Here's how the part is built. I have some questions about the finished solid (model axes, mm). A direction names the side the tool comes from. Give positions to 0.01 mm unless a question says otherwise; leave off trailing zeros. Write each loop counter-clockwise with the first axis right and the second up, starting at its lowest first coordinate (ties: lowest second). Pieces come first, ordered by that corner, then holes. Notation, with made-up numbers: (-15, 52.5) -> (15, 52.5) arc R30 ccw to (15, 79.5) -> close; hole circle Ø1 at (30, -24). An arc over 180 degrees is marked (long way). Use CSV: the item, a comma, the result in double quotes. Start each with the question number.
(1) If we mould it in two halves opening along Y, with no side actions, what happens to faces 3 (the flat face through (-38.1, -26, 0)), 4 (the flat face through (-1, 38.1, 26)), 5 (the flat face through (24, 0, 22.893)), 6 (the flat face through (-25, 0, 22.893))? For each: pulls with the +Y half, pulls with the -Y half, needs draft (parallel to the pull), parting line crosses it, or undercut.
(2) Suppose I cut it at A-A on y = -17.5. List the corners of the cut face in (x, z) for me.
(3) I need wall thicknesses on L1, parallel to Z at x = 1, y = -18.5; L2, parallel to Z at x = 13, y = -9.5; L3, parallel to Y at x = -14, z = -24. Which ranges of each line are inside material? Lowest first, please. Write a range as [from, to].
(4) Which directions (+Z, -Z, +X, -X, +Y, -Y) give clear straight access to the entire face, cutting with the end or side of a thin tool? Please do faces 1 (the flat face through (-1, 0, -27.907)), 2 (the flat face through (0, -1, -38.1)).
(5) Suppose I cut it at C-C on x = 0. List the corners of the cut face in (y, z) for me, plus the area to 3 significant figures.
(6) Suppose I cut it at B-B on z = 0. List the corners of the cut face in (x, y) for me, plus the area to 3 significant figures.
(7) Suppose I cut it at D-D on y = -29.5. List the corners of the cut face in (x, z) for me, plus the area to 3 significant figures.
from build123d import *

# Parameters (mm, degrees)
F0_W     = 76.2
F0_H     = 76.2
F1_DEPTH = 38.1
F2_R     = 25.4
F3_DEPTH = 76.2
F4_R     = 5.08
F5_SIZE  = 5.08
F6_R     = 5.08
F7_R     = 5.08
F8_W     = 50.8
F8_H     = 50.8
F9_DEPTH = 76.2


with BuildPart() as f1:
    # F0 (on Front) → F1 (new body, symmetric)
    with BuildSketch(Plane.XZ):
        Rectangle(F0_W, F0_H)
    extrude(amount=F1_DEPTH, both=True)

    # F2 (on face) → F3 (cut)
    with BuildSketch(Plane.XZ.offset(38.1)):
        Circle(F2_R)
    extrude(amount=-F3_DEPTH, mode=Mode.SUBTRACT)

    # F4
    f4_edges = [f1.edges().sort_by_distance(p)[0] for p in [
        (38.1, 0, 38.1),
    ]]
    fillet(f4_edges, radius=F4_R)

    # F5
    f5_edges = [f1.edges().sort_by_distance(p)[0] for p in [
        (-38.1, 0, 38.1),
    ]]
    chamfer(f5_edges, length=F5_SIZE)

    # F6
    f6_edges = [f1.edges().sort_by_distance(p)[0] for p in [
        (38.1, 0, -38.1),
    ]]
    fillet(f6_edges, radius=F6_R)

    # F7
    f7_edges = [f1.edges().sort_by_distance(p)[0] for p in [
        (-38.1, 0, -38.1),
    ]]
    fillet(f7_edges, radius=F7_R)

    # F8 (on face) → F9 (cut)
    with BuildSketch(Plane(origin=(-38.1, 0, 0), x_dir=(0, -1, 0), z_dir=(-1, 0, 0))):
        with Locations((0, -2.506579)):
            Rectangle(F8_W, F8_H)
    extrude(amount=-F9_DEPTH, mode=Mode.SUBTRACT)


solid = f1.part
Geometry says:
1,face 3,"needs draft"
1,face 4,"pulls with the +Y half"
1,face 5,"undercut"
1,face 6,"undercut"
2,outline,"(-38.1, -33.02) arc R5.08 ccw to (-33.02, -38.1) -> (33.02, -38.1) arc R5.08 ccw to (38.1, -33.02) -> (38.1, -27.91) -> (-38.1, -27.91) -> close; (-38.1, 22.89) -> (-11, 22.89) arc R25.4 cw to (11, 22.89) -> (38.1, 22.89) -> (38.1, 33.02) arc R5.08 ccw to (33.02, 38.1) -> (-33.02, 38.1) -> (-38.1, 33.02) -> close"
3,L1,"[-38.1, -27.91], [25.38, 38.1]"
3,L2,"[-38.1, -27.91], [22.89, 38.1]"
3,L3,"[-38.1, -25.4], [25.4, 38.1]"
4,face 1,"+X, -X"
4,face 2,"-Z, +X, -X, +Y, -Y"
5,outline,"(-38.1, -38.1) -> (38.1, -38.1) -> (38.1, -25.4) -> (25.4, -25.4) -> (25.4, -27.91) -> (-25.4, -27.91) -> (-25.4, -25.4) -> (-38.1, -25.4) -> close; (-38.1, 25.4) -> (38.1, 25.4) -> (38.1, 38.1) -> (-38.1, 38.1) -> close"
5,area,"1,810 mm²"
6,outline,"(-38.1, -38.1) -> (-25.4, -38.1) -> (-25.4, -25.4) -> (-38.1, -25.4) -> close; (-38.1, 25.4) -> (-25.4, 25.4) -> (-25.4, 38.1) -> (-38.1, 38.1) -> close; (25.4, -38.1) -> (38.1, -38.1) -> (38.1, -25.4) -> (25.4, -25.4) -> close; (25.4, 25.4) -> (38.1, 25.4) -> (38.1, 38.1) -> (25.4, 38.1) -> close"
6,area,"645 mm²"
7,outline,"(-38.1, -33.02) arc R5.08 ccw to (-33.02, -38.1) -> (33.02, -38.1) arc R5.08 ccw to (38.1, -33.02) -> (38.1, 33.02) arc R5.08 ccw to (33.02, 38.1) -> (-33.02, 38.1) -> (-38.1, 33.02) -> close; hole circle Ø50.8 at (0, 0)"
7,area,"3,750 mm²"
